Can you work these out from the model? Positions are in its coordinate system, mm. Face numbers are marked on the shaded views. A direction names the side the tool comes from. Coordinates: 2 decimals unless noted, no trailing zeros. Order: outer loops, then holes, each group sorted by start corner. A loop starts at its lowest first (then second) coordinate and runs counter-clockwise, first axis right, second up. Notation, with made-up numbers: (16, 88.25) -> (35, 88.25) arc R16 ccw to (35, 113.25) -> close; hole circle Ø7 at (46.25, 20). An arc over 180 degrees is marked (long way). Answer in a Markdown table with one row per item. Add a question column.
1. Imagine slicing it at B-B on z = -2.56. Write out the boundary of the cut face in (x, y).
2. On a 3-axis mill with a long thin cutter (end or side, diameter ignored), from which of +Z, -Z, +X, -X, +Y, -Y can I reach the whole of each face in a straight line? I mean the marked faces 4, 5 and 6. Say none if no direction works.
3. Imagine slicing it at A-A on y = 0. Write out the boundary of the cut face in (x, z).
4. We'd pull the mould along Z, two halves only. Please class the marked faces 1, 2 and 3: pulls with the +Z half, pulls with the -Z half, needs draft (parallel to the pull), parting line crosses it, or undercut.
5. Imagine slicing it at D-D on y = 5.5. Write out the boundary of the cut face in (x, z), plus the area to 3 significant figures.
6. Will these pins go through, and if not, where does the flat tip stop? pin 1 (8 mm diameter, centred on x = 6.33, y = 0, fed in from -Z); pin 2 (3 mm diameter, centred on x = 15, z = -2.56, fed in from -Y); pin 3 (1.5 mm diameter, centred on x = 15, z = -2.5, fed in from +Y).
7. If I drill on line 1 along X through (y, z) = (-1.25, -2.5); line 2 along Y through (x, z) = (13.75, -2.65); line 3 along Z through (x, y) = (11.25, 2.5), over which ranges is the centre line in solid material (lowest first)? Write a range as [from, to].
8. Imagine slicing it at C-C on x = 13.75. Write out the boundary of the cut face in (y, z).
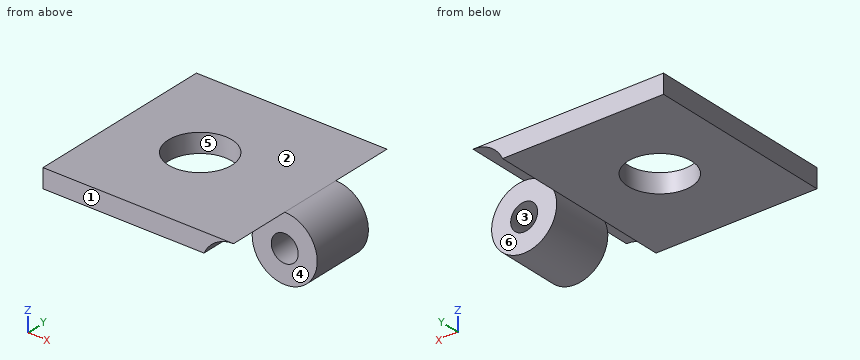
from build123d import *

# Parameters (mm, degrees)
BOSS_EXTRUDE1_DEPTH      = 7.5
BOSS_EXTRUDE1_DEPTH_BACK = 7.5
BOSS_EXTRUDE3_DEPTH      = 2.5
BOSS_EXTRUDE3_DEPTH_BACK = 2.5
SKETCH1_4_R              = 2.56
SKETCH1_4_R_2            = 1.06
SKETCH2_R                = 2.5
CUT_EXTRUDE1_DEPTH       = 3


with BuildPart() as part:
    # Sketch1 → Boss-Extrude1 (new, two sides: drawn at the far end of the back side and taken through both)
    with BuildSketch(Plane(origin=(0, 0, 0), x_dir=(1, 0, 0), z_dir=(0, 1, 0)).offset(-BOSS_EXTRUDE1_DEPTH_BACK)):
        with BuildLine():
            Line((0, 1.5), (0, 0))
            Line((0, 0), (15, 0))
            ThreePointArc((15, 0), (13.614359354, 0.407420152), (12.66976396, 1.5))
            Line((12.66976396, 1.5), (0, 1.5))
        make_face()
    extrude(amount=BOSS_EXTRUDE1_DEPTH + BOSS_EXTRUDE1_DEPTH_BACK)

    # Sketch1_4 → Boss-Extrude3 (add, two sides: drawn at the far end of the back side and taken through both)
    with BuildSketch(Plane(origin=(0, 0, 0), x_dir=(1, 0, 0), z_dir=(0, 1, 0)).offset(-BOSS_EXTRUDE3_DEPTH_BACK)):
        with Locations((15, 2.56)):
            Circle(SKETCH1_4_R)
        with Locations(Location((15, 2.56, 0), (0, 0, 270))):
            Circle(SKETCH1_4_R_2, mode=Mode.SUBTRACT)
    extrude(amount=BOSS_EXTRUDE3_DEPTH + BOSS_EXTRUDE3_DEPTH_BACK)

    # Sketch2 → Cut-Extrude1 (cut)
    with BuildSketch(Plane(origin=(0, 0, -1.5), x_dir=(-1, 0, 0), z_dir=(0, 0, -1))):
        with Locations((-6.33488198, 0)):
            Circle(SKETCH2_R)
    extrude(amount=-CUT_EXTRUDE1_DEPTH, mode=Mode.SUBTRACT)


solid = part.part
Answers follow:
| question | item | result |
|---|---|---|
| 1 | outline | (12.44, -2.5) -> (13.94, -2.5) -> (13.94, 2.5) -> (12.44, 2.5) -> close; (16.06, -2.5) -> (17.56, -2.5) -> (17.56, 2.5) -> (16.06, 2.5) -> close |
| 2 | face 4 | -Z, +X, -Y |
| 2 | face 5 | +Z, -Z |
| 2 | face 6 | -Z, +X, +Y |
| 3 | outline | (0, -1.5) -> (3.83, -1.5) -> (3.83, 0) -> (0, 0) -> close; (8.83, -1.5) -> (12.67, -1.5) arc R2.56 ccw (long way) to (15, 0) -> (8.83, 0) -> close; hole circle Ø2.12 at (15, -2.56) |
| 4 | face 1 | needs draft |
| 4 | face 2 | pulls with the +Z half |
| 4 | face 3 | undercut |
| 5 | outline | (0, -1.5) -> (12.67, -1.5) arc R2.56 cw to (15, 0) -> (0, 0) -> close |
| 5 | area | 20.0 mm² |
| 6 | pin 1 | stops at z = -1.5 |
| 6 | pin 2 | stops at y = -2.5 |
| 6 | pin 3 | passes through |
| 7 | line 1 | x = [12.44, 13.94], [16.06, 17.56] |
| 7 | line 2 | y = [-2.5, 2.5] |
| 7 | line 3 | z = [-1.5, 0] |
| 8 | outline | (-7.5, -0.33) -> (-2.5, -0.33) -> (-2.5, -4.79) -> (2.5, -4.79) -> (2.5, -0.33) -> (7.5, -0.33) -> (7.5, 0) -> (-7.5, 0) -> close |
